Part model, mm, in its own coordinate system. A direction names the side the tool comes from. Coordinates: 2 decimals unless noted, no trailing zeros. Loops run counter-clockwise (first coordinate to the right, second up) from the corner with the lowest first, then second, coordinate; pieces in that order, holes last. Notation, with made-up numbers: (-26, 80.25) - (-20, 80.25) arc R21 cw to (-20, 98.25) - close; hole circle Ø5 at (31, -3.5). An arc over 180 degrees is marked (long way). Use a Markdown table: item, result. Add a question column.
1) Band-saw the part on C-C (x = 3.5). Give the cut face in (y, z).
2) Tool access for faces 1 (the face through (59, -131, 0)), 2 (the face through (0, -100, 12)): list every direction of +Z, -Z, +X, -X, +Y, -Y with a clear straight run to the whole face (end or side of a thin tool).
3) Pull direction Y, two halves, no side cores. Call faces 3 (the face through (2, 0, 19)), 4 (the face through (2, -266, 19)), 5 (the face through (30.271, -133, 12)), 6 (the face through (-129.358, -131, 19)): +Y half, -Y half, draft (parallel to the pull), parting line (faces both ways), or undercut.
4) Band-saw the part on A-A (y = -105). Give the cut face in (x, z), plus the area to 3 significant figures.
5) Drop flat-ended pins along their axis: P1, Ø10, axis at y = -205.5, z = 4, coming from the +X side; P2, Ø18, axis at x = 1, y = -140.5, coming from the -Z side. Give the stop position or say it passes through.
6) Probe probe 1 along Y at (x, z) = (29, 13); probe 2 along X at (y, z) = (-160.5, 6); probe 3 along X at (y, z) = (-85, 3.5). List the from-to ranges inside material, lowest first. Write a range as [from, to].
7) Band-saw the part on B-B (z = 13.5). Give the cut face in (x, y), plus the area to 3 significant figures.
from build123d import *

# Parameters (mm, degrees)
F0_W     = 266
F0_H     = 33.3
F1_DEPTH = 266
F2_W     = 60.54271
F2_H     = 66
F3_DEPTH = 25
F4_SIZE  = 5


with BuildPart() as f1:
    # F0 (on Front) → F1 (new body)
    with BuildSketch(Plane.XZ):
        with Locations((3.64231, 16.65)):
            Rectangle(F0_W, F0_H)
    extrude(amount=F1_DEPTH)

    # F2 (on face) → F3 (cut)
    with BuildSketch(Plane(origin=(0, 0, 0), x_dir=(1, 0, 0), z_dir=(0, 0, -1))):
        with Locations((0, 133)):
            Rectangle(F2_W, F2_H)
    extrude(amount=-F3_DEPTH, mode=Mode.SUBTRACT)

    # F4
    f4_edges = [f1.edges().sort_by_distance(p)[0] for p in [
        (136.64231, -266, 16.65),
        (136.64231, 0, 16.65),
        (-129.35769, 0, 16.65),
        (-129.35769, -266, 16.65),
        (-129.35769, -133, 0),
        (3.64231, -266, 0),
        (136.64231, -133, 0),
        (3.64231, 0, 0),
    ]]
    chamfer(f4_edges, length=F4_SIZE)


solid = f1.part
Answer block:
| question | item | result |
|---|---|---|
| 1 | outline | (-266, 5) - (-261, 0) - (-166, 0) - (-166, 25) - (-100, 25) - (-100, 0) - (-5, 0) - (0, 5) - (0, 33.3) - (-266, 33.3) - close |
| 2 | face 1 | -Z, +X, -X, +Y, -Y |
| 2 | face 2 | -Z |
| 3 | face 3 | +Y half |
| 3 | face 4 | -Y half |
| 3 | face 5 | undercut |
| 3 | face 6 | draft |
| 4 | outline | (-129.36, 5) - (-124.36, 0) - (-30.27, 0) - (-30.27, 25) - (30.27, 25) - (30.27, 0) - (131.64, 0) - (136.64, 5) - (136.64, 33.3) - (-129.36, 33.3) - close |
| 4 | area | 7,320 mm2 |
| 5 | P1 | x = 136.64 |
| 5 | P2 | z = 25 |
| 6 | probe 1 | [-266, -166], [-100, 0] |
| 6 | probe 2 | [-129.36, -30.27], [30.27, 136.64] |
| 6 | probe 3 | [-127.86, 135.14] |
| 7 | outline | (-129.36, -261) - (-124.36, -266) - (131.64, -266) - (136.64, -261) - (136.64, -5) - (131.64, 0) - (-124.36, 0) - (-129.36, -5) - close; hole (-30.27, -166) - (30.27, -166) - (30.27, -100) - (-30.27, -100) - close |
| 7 | area | 66,700 mm2 |
